Design review of the part shown in the three views and the two pictorial views. Dimensions are in mm from the part's minimum x, y and z. Coordinates: 2 decimals unless noted, no trailing zeros. Write each loop counter-clockwise with the first axis right and the second up, starting at its lowest first coordinate (ties: lowest second). Pieces come first, ordered by that corner, then holes. Notation, with made-up numbers: (45, 7.25) - (81, 7.25) arc R18 ccw to (81, 33.25) - close; hole circle Ø9 at (-29.75, 51). An arc over 180 degrees is marked (long way). Answer as CSV lines item,"result". Start each with the question number.
Q1. Clearance check with flat-ended pins moving along their axes: pin 1 (2 mm diameter, centred on x = 3.5, z = 3, fed in from -Y); pin 2 (3 mm diameter, centred on x = 5, z = 19.5, fed in from +Y); pin 3 (1.5 mm diameter, centred on x = 3, y = 3.46, fed in from -Z); pin 4 (3 mm diameter, centred on x = 3, z = 18.5, fed in from +Y). State where each tip first meets the part, or that it passes through.
Q2. We need section A-A (z = 22). Write out the cut boundary in (x, y).
Q3. For line 1 along Y through (x, z) = (3.4, 2); line 2 along X through (y, z) = (4.5, 25); line 3 along X through (y, z) = (3.25, 15.5), list the stretches that pass through material, from the lowest coordinate up. Write a range as [from, to].
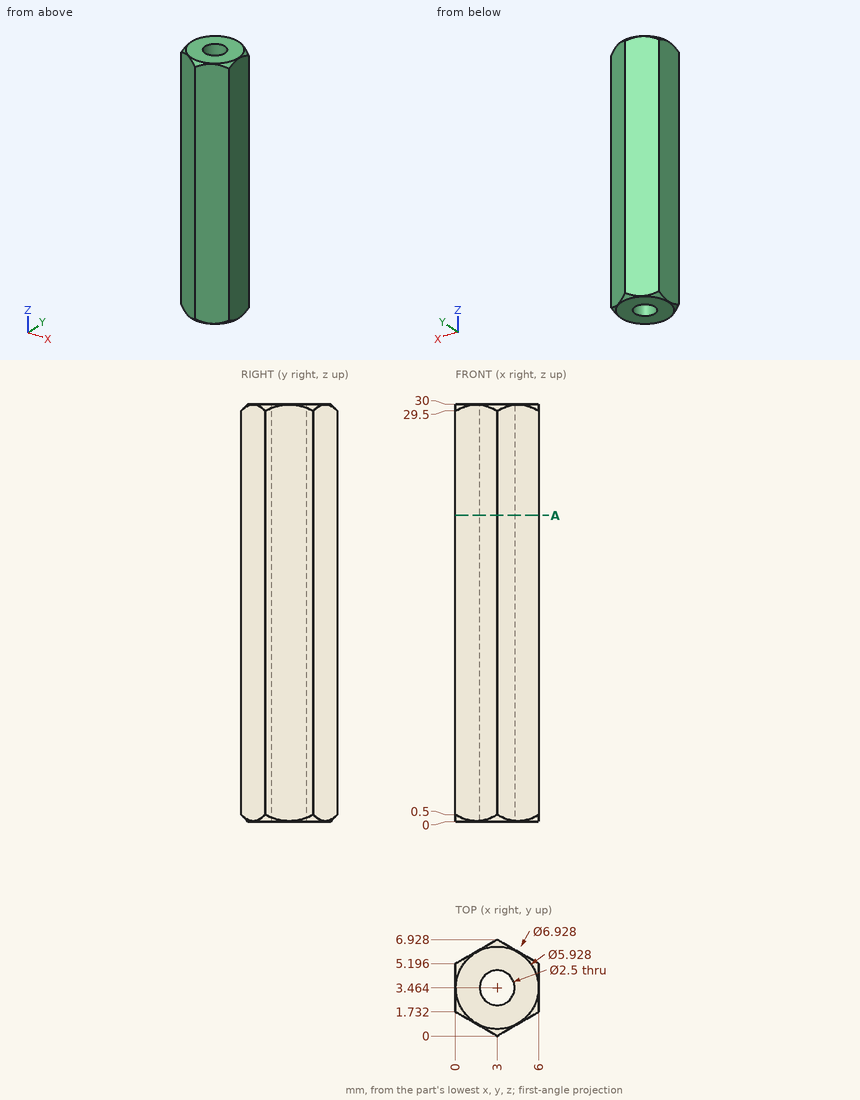
Results list:
1,pin 1,"stops at y = 0"
1,pin 2,"stops at y = 6.64"
1,pin 3,"passes through"
1,pin 4,"stops at y = 6.93"
2,outline,"(0, 1.73) - (3, 0) - (6, 1.73) - (6, 5.2) - (3, 6.93) - (0, 5.2) - close; hole circle Ø2.5 at (3, 3.46)"
3,line 1,"y = [0.23, 2.28], [4.65, 6.7]"
3,line 2,"x = [0, 2.3], [3.7, 6]"
3,line 3,"x = [0, 1.77], [4.23, 6]"
